Can you work these out from the model? Positions are in its coordinate system, mm. A direction names the side the tool comes from. Give positions to 0.01 mm unless a question says otherwise; leave off trailing zeros. Order: outer loops, then holes, each group sorted by start corner. A loop starts at its lowest first (then second) coordinate and runs counter-clockwise, first axis right, second up. Notation, with made-up numbers: (-16.75, 80) - (16.25, 80) arc R12 ccw to (16.25, 94) - close; hole circle Ø11 at (10.5, 12). An arc over 180 degrees is marked (long way). Use one line per item in the form item = value. Start each with the question number.
1) Which directions (+Z, -Z, +X, -X, +Y, -Y) give clear straight access to the entire face, cutting with the end or side of a thin tool? Please do faces 1 (the cylindrical face through (-44.848, -34.388, 0.27)), 2 (the cylindrical face through (-12.035, 54.195, 21.976)), 3 (the flat face through (51.288, 30.167, 29.142)).
2) Suppose I cut it at C-C, the plane z = 30.5. Write out the boundary of the cut face in (x, y).
3) Please list where these lines run through material, in increasing order: probe 1 along Y at (x, z) = (-1.5, -2.5); probe 2 along X at (y, z) = (-27, -15); probe 3 along Y at (x, z) = (28.5, -14.5).
4) Suppose I cut it at B-B, the plane z = 14.5. Write out the boundary of the cut face in (x, y) (3 decimals), and give its area (3 significant figures).
5) Suppose I cut it at A-A, the plane x = 0. Write out the boundary of the cut face in (y, z) (3 decimals).
6) For pin 1 (10 mm diameter, centred on x = 43, z = 23.5, fed in from +Y); pin 2 (3 mm diameter, centred on x = 43, z = 8.5, fed in from +Y); pin 3 (4 mm diameter, centred on x = -3, z = -13.5, fed in from +Y); pin 4 (10 mm diameter, centred on x = 39, z = 22, fed in from +Y), each with a flat end and sliding along its axis, tell me the tip position at first contact or that it passes through.
Autodesk Inventor part; units mm, degrees
ref_plane "YZ Plane" through (0, 0, 0) normal (1, 0, 0) x (0, 1, 0)
ref_plane "XZ Plane" through (0, 0, 0) normal (0, 1, 0) x (-1, 0, 0)
ref_plane "XY Plane" through (0, 0, 0) normal (0, 0, 1) x (1, 0, 0)
sketch "Szkic7" plane through (0, 0, 0) normal (0, 0, 1) x (1, 0, 0)
  circle A0 centre (0, 0) radius 56.515
  dimension "d35" = 113.03
extrude "Wyciągnięcie proste2" add sketch "Szkic7" along normal mid plane 40.5625
chamfer "Faza2" distance 1 angle 45 1 edges at (-56.515, 0, 20.2812)
sketch "Szkic9" plane through (0, 0, 20.2812) normal (0, 0, 1) x (1, 0, 0)
  circle A0 centre (0, 0) radius 55.515
extrude "Wyciągnięcie proste3" add sketch "Szkic9" along normal blind 3.4375
sketch "Szkic10" plane through (0, 0, 23.7188) normal (0, 0, 1) x (1, 0, 0)
  line L0 (-34.3523, 59.5) -> (34.3523, 59.5)
  line L1 (34.3523, 59.5) -> (68.7047, 0)
  line L2 (68.7047, 0) -> (34.3523, -59.5)
  line L3 (34.3523, -59.5) -> (-34.3523, -59.5)
  line L4 (-34.3523, -59.5) -> (-68.7047, 0)
  line L5 (-68.7047, 0) -> (-34.3523, 59.5)
  line L6 (0, 79.121) -> (0, -79.121) construction
  line L7 (-79.121, 0) -> (79.121, 0) construction
  point P0 (0, 0)
  point P1 (0, 0)
  point P2 (0, 59.5)
  dimension "d44" = 119
extrude "Wyciągnięcie proste4" add sketch "Szkic10" along normal blind 11
sketch "Szkic12" plane through (0, 0, 0) normal (0, 1, 0) x (-1, 0, 0)
  line L0 (0, -2.1463) -> (0, 12.8775) construction
  line L1 (-34.3523, 23.7188) -> (-34.3523, 34.7188) construction
  line L2 (-68.7047, 34.7188) -> (-34.3523, 34.7188) construction
  line L3 (-68.7047, 23.7188) -> (-68.7047, 34.7188)
  line L4 (-68.7047, 32.593) -> (-60.7713, 34.7188)
  line L5 (-68.7047, 34.7188) -> (-34.3523, 34.7188)
  line L6 (-68.7047, 23.7188) -> (-34.3523, 23.7188)
  point P0 (0, 0)
  dimension "d50" = 15
  dimension "d51" = 7.9333
revolve "Obrót2" cut sketch "Szkic12" angle 360 about axis through (0, 0, -10) along (0, 0, 1)
thread "Gwint3"
chamfer "Faza3" distance 1 angle 45 1 edges at (-56.515, 0, -20.2812)
equation "\"d35\" = OD"
equation "\"d36\" = 0.7375 * L"
equation "\"d42\" = 0.0625 * L"
equation "\"d44\" = SW"
equation "\"d45\" = 0.2 * L"
equation "\"d51\" = 0.0666667 * SW"
equation "\"SzerokośćGięciaPodcięcia\" = Grubość"
equation "\"RozmiarPodcięciaNarożnika\" = 4 * Grubość"
equation "\"PromieńPrzejścia\" = PromieńGięcia"
equation "\"Rozmiar_promienia_Jacobiego\" = PromieńGięcia"
equation "\"Wielk_odstępu\" = Grubość"
equation "\"d2\" = PromieńGięcia"
equation "\"d23\" = PromieńGięcia"
equation "\"OD\" = 113.03"
equation "\"SW\" = 119"
equation "\"L\" = 55"
properties part number "Korek sześciokątny BSP 4'' L=55" material "304"
Result sheet:
q1.face_1 = -Z
q1.face_2 = none
q1.face_3 = +Z, -Z, +X, +Y
q2.outline = (-68.7, 0) - (-34.35, -59.5) - (34.35, -59.5) - (68.7, 0) - (34.35, 59.5) - (-34.35, 59.5) - close
q3.probe_1 = -56.5 to 56.5
q3.probe_2 = -49.65 to 49.65
q3.probe_3 = -48.8 to 48.8
q4.outline = circle Ø113.03 at (0, 0)
q4.area = 10,000 mm²
q5.outline = (-59.5, 23.719) - (-55.515, 23.719) - (-55.515, 20.281) - (-56.515, 19.281) - (-56.515, -19.281) - (-55.515, -20.281) - (55.515, -20.281) - (56.515, -19.281) - (56.515, 19.281) - (55.515, 20.281) - (55.515, 23.719) - (59.5, 23.719) - (59.5, 34.719) - (-59.5, 34.719) - close
q6.pin_1 = 53.17
q6.pin_2 = 38.36
q6.pin_3 = 56.51
q6.pin_4 = 59.5
